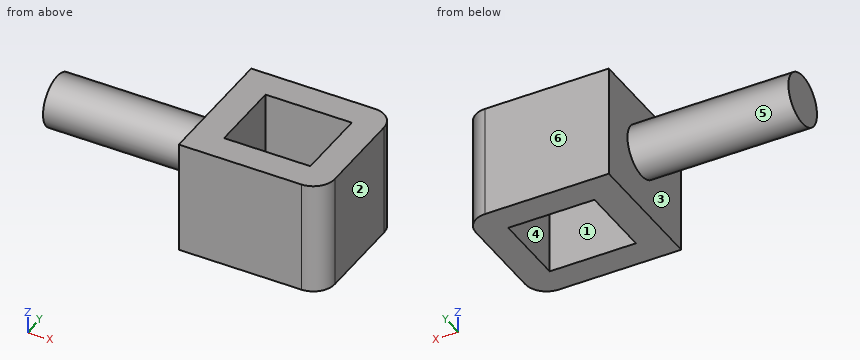
```python
from build123d import *

# Parameters (mm, degrees)
F0_W     = 94.618846
F0_H     = 85.351713
F1_DEPTH = 74.324219
F2_W     = 56.600913
F2_H     = 48.861958
F3_DEPTH = 132.836582
F4_R     = 16.833505
F5_DEPTH = 105.622353
F6_R     = 14.149732
F7_R     = 13.33873


with BuildPart() as f1:
    # F0 (on Top) → F1 (new body)
    with BuildSketch(Plane.XY):
        with Locations((3.090644, -3.800507)):
            Rectangle(F0_W, F0_H)
    extrude(amount=F1_DEPTH)

    # F2 (on face) → F3 (cut)
    with BuildSketch(Plane.XY.offset(74.324219)):
        with Locations((3.696986, -3.887054)):
            Rectangle(F2_W, F2_H)
    extrude(amount=-F3_DEPTH, mode=Mode.SUBTRACT)

    # F4 (on face) → F5 (join)
    with BuildSketch(Plane(origin=(-44.218779, 0, 0), x_dir=(0, -1, 0), z_dir=(-1, 0, 0))):
        with Locations((0, 39.672762)):
            Circle(F4_R)
    extrude(amount=F5_DEPTH)

    # F6
    f6_edges = [f1.edges().sort_by_distance(p)[0] for p in [
        (50.400067, -46.476364, 37.162109),
    ]]
    fillet(f6_edges, radius=F6_R)

    # F7
    f7_edges = [f1.edges().sort_by_distance(p)[0] for p in [
        (50.400067, 38.875349, 37.162109),
    ]]
    fillet(f7_edges, radius=F7_R)


solid = f1.part
```
Check sheet for the modelled part. Datum: model origin and axes. Units: mm. Face numbers are marked on the shaded views. A direction names the side the tool comes from. Round coordinates to 2 decimals unless told otherwise and drop trailing zeros. Loops run counter-clockwise (first coordinate to the right, second up) from the corner with the lowest first, then second, coordinate; pieces in that order, holes last. Notation, with made-up numbers: M 45,33.25 L 59,33.25 A35 cw 59,68.25 Z; hole C 4.25,85.5 d1. An arc over 180 degrees is marked long. Answer as a JSON object with one key per item and string values.
1. Section check B-B (y = 0). Record the boundary of the cut face in (x, z).
Reply:
{"outline": "M -149.84,22.84 L -44.22,22.84 L -44.22,0 L -24.6,0 L -24.6,74.32 L -44.22,74.32 L -44.22,56.51 L -149.84,56.51 Z; M 32,0 L 50.4,0 L 50.4,74.32 L 32,74.32 Z"}
2. Scan lines: line 1 (X direction, y = -11.5, z = 26.5); line 2 (Y direction, x = 10, z = 40.5); line 3 (X direction, y = 13.5, z = 49). Record each from-to range of solid material in increasing order.
Reply:
{"line 1": "x = -44.22 to -24.6, 32 to 50.4", "line 2": "y = -46.48 to -28.32, 20.54 to 38.88", "line 3": "x = -149.84 to -24.6, 32 to 50.4"}
3. Gauge pin test, flat ends, axial feed: P1, Ø3, axis at x = -123.5, y = -1, coming from the -Z side; P2, Ø6, axis at x = -59, z = 51.5, coming from the +Y side; P3, Ø6, axis at y = -34.5, z = 9, coming from the -X side; P4, Ø4, axis at x = -122.5, y = -19, coming from the +Z side. Record the tip position at first contact, or that the pin passes through.
Reply:
{"P1": "stops at z = 22.84", "P2": "stops at y = 14.33", "P3": "stops at x = -44.22", "P4": "passes through"}
4. Section check C-C (z = 65.5). Record the boundary of the cut face in (x, y), plus the area to 3 significant figures.
Reply:
{"outline": "M -44.22,-46.48 L 36.25,-46.48 A14.15 ccw 50.4,-32.33 L 50.4,25.54 A13.34 ccw 37.06,38.88 L -44.22,38.88 Z; hole M -24.6,-28.32 L 32,-28.32 L 32,20.54 L -24.6,20.54 Z", "area": "5,230 mm²"}
5. Section check A-A (x = 21.5). Record the boundary of the cut face in (y, z).
Reply:
{"outline": "M -46.48,0 L -28.32,0 L -28.32,74.32 L -46.48,74.32 Z; M 20.54,0 L 38.88,0 L 38.88,74.32 L 20.54,74.32 Z"}
6. Section check D-D (z = 34). Record the boundary of the cut face in (x, y), plus the area to 3 significant figures.
Reply:
{"outline": "M -149.84,-15.85 L -44.22,-15.85 L -44.22,-46.48 L 36.25,-46.48 A14.15 ccw 50.4,-32.33 L 50.4,25.54 A13.34 ccw 37.06,38.88 L -44.22,38.88 L -44.22,15.85 L -149.84,15.85 Z; hole M -24.6,-28.32 L 32,-28.32 L 32,20.54 L -24.6,20.54 Z", "area": "8,580 mm²"}
7. Access from +Z, -Z, +X, -X, +Y, -Y to the whole of each face (thin tool, end or side, straight path). Record for the marked faces 1, 2 and 3.
Reply:
{"face 1": "+Z, -Z", "face 2": "+Z, -Z, +X, +Y, -Y", "face 3": "-X"}
8. Mould release check, pull along Y, two halves, no side actions. Record for the marked faces 4, 5 and 6: pulls with the +Y half, pulls with the -Y half, needs draft (parallel to the pull), parting line crosses it, or undercut.
Reply:
{"face 4": "undercut", "face 5": "parting line crosses it", "face 6": "pulls with the +Y half"}
